Build history of the part. All positions in model axes, mm. Face numbers are marked on the shaded views. A direction names the side the tool comes from. Give positions to 0.01 mm unless a question says otherwise; leave off trailing zeros. Write each loop counter-clockwise with the first axis right and the second up, starting at its lowest first coordinate (ties: lowest second). Pieces come first, ordered by that corner, then holes.
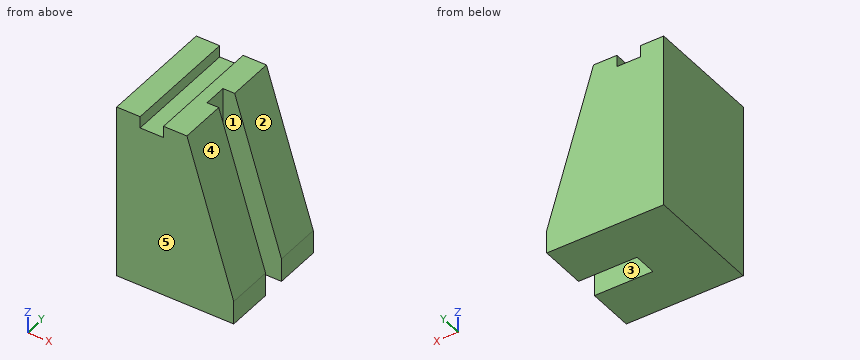
from build123d import *

# Parameters (mm, degrees)
F1_DEPTH = 100
F4_DEPTH = 150
F5_DEPTH = 100


with BuildPart() as f1:
    # F0 (on Front) → F1 (new body)
    with BuildSketch(Plane.XZ):
        Polygon((0, 150), (0, 0), (100, 0), (100, 20), (60, 150), (40, 150), (40, 140), (20, 140), (20, 150), align=None)
    extrude(amount=F1_DEPTH)

    # F3 (on face) → F4 (cut)
    with BuildSketch(Plane.XY.offset(150)):
        Polygon((60, -60), (60, -50), (60, -40), (50, -40), (50, -60), align=None)
    extrude(amount=-F4_DEPTH, mode=Mode.SUBTRACT)

    # F5 (cut): a face of the model
    f5_faces = [f1.faces().sort_by_distance(p)[0] for p in [
        (60, -50, 75),
    ]]
    extrude(f5_faces, amount=-F5_DEPTH, mode=Mode.SUBTRACT)


solid = f1.part
1. Saw through at B-B on y = -27. Give the cut face in (x, z), plus the area to 3 significant figures.
2. Saw through at D-D on x = 82. Give the cut face in (y, z), plus the area to 3 significant figures.
3. Mould opens along Y. For the marked faces 3, 4 and 5 say: pulls with the +Y half, pulls with the -Y half, needs draft (parallel to the pull), parting line crosses it, or undercut.
4. Drop flat-ended pins along their axis: pin 1 (10 mm diameter, centred on y = -49.5, z = 112, fed in from +X); pin 2 (4 mm diameter, centred on y = -24.5, z = 99.5, fed in from +X); pin 3 (6 mm diameter, centred on x = 26, y = -46.5, fed in from +Z). Give the stop position or say it passes through.
5. Saw through at A-A on x = 66. Give the cut face in (y, z).
6. 3-axis set-ups, long thin cutter, end or side, ignore diameter. For the marked faces 1 and 2: which of +Z, -Z, +X, -X, +Y, -Y reach the whole face in a straight line?
7. Saw through at C-C on z = 115.5. Give the cut face in (x, y).
8. Drill centre lines: line 1 along Y through (x, z) = (70, 48.5); line 2 along X through (y, z) = (-40.5, 64.5); line 3 along Z through (x, y) = (36.5, -72). Where is each one in solid material? Low to high.
Outcome:
1. outline: (0, 0) - (100, 0) - (100, 20) - (60, 150) - (40, 150) - (40, 140) - (20, 140) - (20, 150) - (0, 150) - close
1. area: 12,200 mm2
2. outline: (-100, 0) - (-60, 0) - (-60, 78.5) - (-100, 78.5) - close; (-40, 0) - (0, 0) - (0, 78.5) - (-40, 78.5) - close
2. area: 6,280 mm2
3. face 3: undercut
3. face 4: needs draft
3. face 5: pulls with the -Y half
4. pin 1: stops at x = 50
4. pin 2: stops at x = 76.15
4. pin 3: stops at z = 140
5. outline: (-100, 0) - (-60, 0) - (-60, 130.5) - (-100, 130.5) - close; (-40, 0) - (0, 0) - (0, 130.5) - (-40, 130.5) - close
6. face 1: +Z, -Z, +X
6. face 2: +Z, +X, +Y, -Y
7. outline: (0, -100) - (70.62, -100) - (70.62, -60) - (50, -60) - (50, -40) - (70.62, -40) - (70.62, 0) - (0, 0) - close
8. line 1: y = -100 to -60, -40 to 0
8. line 2: x = 0 to 50
8. line 3: z = 0 to 140
